from build123d import *

# Parameters (mm, degrees)
BOSS_EXTRUDE1_DEPTH  = 5
FILLET1_R            = 1
BOSS_EXTRUDE17_DEPTH = 7
CHAMFER1_SIZE        = 6
CHAMFER2_SIZE        = 6
CHAMFER3_SIZE        = 6


with BuildPart() as part:
    # Sketch2 → Boss-Extrude1 (new body)
    with BuildSketch(Plane.XY):
        with BuildLine():
            Line((-71.683238322, 36.264064839), (-71.683238322, -153.735935161))
            ThreePointArc((-71.683238322, -153.735935161), (-65.785654561, -167.973961861), (-51.547627861, -173.871545622))
            ThreePointArc((-51.547627861, -173.871545622), (38.452372139, -179.984063939), (128.452372139, -173.871545622))
            ThreePointArc((128.452372139, -173.871545622), (142.690398839, -167.973961861), (148.5879826, -153.735935161))
            Line((148.5879826, -153.735935161), (148.5879826, 36.264064839))
            ThreePointArc((148.5879826, 36.264064839), (146.404575746, 42.501121163), (140.807808283, 46.014571182))
            ThreePointArc((140.807808283, 46.014571182), (138.971586139, 46.086284232), (137.233469629, 45.489789872))
            ThreePointArc((137.233469629, 45.489789872), (38.452372139, 19.454880614), (-60.328725351, 45.489789872))
            ThreePointArc((-60.328725351, 45.489789872), (-62.066841861, 46.086284232), (-63.903064005, 46.014571182))
            ThreePointArc((-63.903064005, 46.014571182), (-69.499831468, 42.501121163), (-71.683238322, 36.264064839))
        make_face()
        with BuildLine():
            Line((-51.547627861, -162.258832658), (128.989007395, -162.258832658))
            ThreePointArc((128.989007395, -162.258832658), (131.022308029, -167.563941455), (126.782256855, -171.345535941))
            ThreePointArc((126.782256855, -171.345535941), (38.682041526, -176.831727196), (-49.421685934, -171.402229683))
            ThreePointArc((-49.421685934, -171.402229683), (-53.676249609, -167.572612121), (-51.547627861, -162.258832658))
        make_face(mode=Mode.SUBTRACT)
    extrude(amount=BOSS_EXTRUDE1_DEPTH)

    # Fillet1
    fillet1_edges = [part.edges().sort_by_distance(p)[0] for p in [
        (38.452372139, 19.454880614, 5),
        (38.452372139, -179.984063939, 0),
        (-65.785654561, -167.973961861, 0),
        (-71.683238322, -58.735935161, 0),
        (-69.499831468, 42.501121163, 0),
        (-62.066841861, 46.086284232, 0),
        (38.452372139, 19.454880614, 0),
        (138.971586139, 46.086284232, 0),
        (146.404575746, 42.501121163, 0),
        (-62.066841861, 46.086284232, 5),
        (-69.499831468, 42.501121163, 5),
        (128.452372139, -173.871545622, 2.5),
        (-51.547627861, -173.871545622, 2.5),
        (-71.683238322, -58.735935161, 5),
        (-65.785654561, -167.973961861, 5),
        (38.452372139, -179.984063939, 5),
        (142.690398839, -167.973961861, 5),
        (148.5879826, -58.735935161, 5),
        (146.404575746, 42.501121163, 5),
        (138.971586139, 46.086284232, 5),
        (148.5879826, -58.735935161, 0),
        (142.690398839, -167.973961861, 0),
    ]]
    fillet(fillet1_edges, radius=FILLET1_R)

    # Sketch3 → Boss-Extrude17 (add)
    with BuildSketch(Plane(origin=(0, 0, 0), x_dir=(-1, 0, 0), z_dir=(0, 0, -1))):
        Polygon((-60.193398692, -12.441134496), (-80.193398692, -23.98813988), (-80.193398692, -47.082150648), (-60.193398692, -58.629156031), (-40.193398692, -47.082150648), (-40.193398692, -23.98813988), align=None)
        Polygon((-39.260340262, -48.416474981), (-59.281974378, -59.975970827), (-59.281974378, -83.094962521), (-39.260340262, -94.654458367), (-19.238706146, -83.094962521), (-19.238706146, -59.975970827), align=None)
        Polygon((-59.655195417, -84.642570383), (-79.655195417, -96.189575767), (-79.655195417, -119.283586535), (-59.655195417, -130.830591919), (-39.655195417, -119.283586535), (-39.655195417, -96.189575767), align=None)
        Polygon((-18.449927197, -84.144928283), (-38.449927197, -95.691933667), (-38.449927197, -118.785944435), (-18.449927197, -130.332949819), (1.550072803, -118.785944435), (1.550072803, -95.691933667), align=None)
        Polygon((2.303708649, -48.596386935), (-17.696291351, -60.143392319), (-17.696291351, -83.237403087), (2.303708649, -94.78440847), (22.303708649, -83.237403087), (22.303708649, -60.143392319), align=None)
        Polygon((-80.491202658, -48.737511822), (-100.491202658, -60.284517205), (-100.491202658, -83.378527973), (-80.491202658, -94.925533357), (-60.491202658, -83.378527973), (-60.491202658, -60.284517205), align=None)
        Polygon((-18.755317237, -12.540627892), (-38.755317237, -24.087633275), (-38.755317237, -47.181644043), (-18.755317237, -58.728649427), (1.244682763, -47.181644043), (1.244682763, -24.087633275), align=None)
    extrude(amount=BOSS_EXTRUDE17_DEPTH)

    # Chamfer1
    chamfer1_edges = [part.edges().sort_by_distance(p)[0] for p in [
        (70.491202658, -54.511014514, -7),
        (90.491202658, -54.511014514, -7),
        (100.491202658, -71.831522589, -7),
        (90.491202658, -89.152030665, -7),
        (70.491202658, -89.152030665, -7),
        (60.491202658, -71.831522589, -7),
    ]]
    chamfer(chamfer1_edges, length=CHAMFER1_SIZE)

    # Chamfer2
    chamfer2_edges = [part.edges().sort_by_distance(p)[0] for p in [
        (-12.303708649, -54.369889627, -7),
        (7.696291351, -54.369889627, -7),
        (17.696291351, -71.690397703, -7),
        (7.696291351, -89.010905779, -7),
        (-12.303708649, -89.010905779, -7),
        (-22.303708649, -71.690397703, -7),
    ]]
    chamfer(chamfer2_edges, length=CHAMFER2_SIZE)

    # Chamfer3
    chamfer3_edges = [part.edges().sort_by_distance(p)[0] for p in [
        (50.193398692, -18.214637188, -7),
        (70.193398692, -18.214637188, -7),
        (80.193398692, -35.535145264, -7),
        (70.193398692, -52.855653339, -7),
        (50.193398692, -52.855653339, -7),
        (40.193398692, -35.535145264, -7),
        (29.249523204, -54.196222904, -7),
        (49.27115732, -54.196222904, -7),
        (59.281974378, -71.535466674, -7),
        (49.27115732, -88.874710444, -7),
        (29.249523204, -88.874710444, -7),
        (19.238706146, -71.535466674, -7),
        (49.655195417, -90.416073075, -7),
        (69.655195417, -90.416073075, -7),
        (79.655195417, -107.736581151, -7),
        (69.655195417, -125.057089227, -7),
        (49.655195417, -125.057089227, -7),
        (39.655195417, -107.736581151, -7),
        (8.449927197, -89.918430975, -7),
        (28.449927197, -89.918430975, -7),
        (38.449927197, -107.238939051, -7),
        (28.449927197, -124.559447127, -7),
        (8.449927197, -124.559447127, -7),
        (-1.550072803, -107.238939051, -7),
        (8.755317237, -18.314130583, -7),
        (28.755317237, -18.314130583, -7),
        (38.755317237, -35.634638659, -7),
        (28.755317237, -52.955146735, -7),
        (8.755317237, -52.955146735, -7),
        (-1.244682763, -35.634638659, -7),
    ]]
    chamfer(chamfer3_edges, length=CHAMFER3_SIZE)


solid = part.part
Build history of the part. All positions in model axes, mm. A direction names the side the tool comes from. Coordinates: 2 decimals unless noted, no trailing zeros. Order: outer loops, then holes, each group sorted by start corner. A loop starts at its lowest first (then second) coordinate and runs counter-clockwise, first axis right, second up. Notation, with made-up numbers: (-19, 8.5) - (-12, 8.5) arc R27 ccw to (-12, 38.5) - close; hole circle Ø5 at (86, 58). An arc over 180 degrees is marked (long way). Write each question's results on one line, items separated by ' | '. Start each with the question number.
Item 1: Band-saw the part on B-B on z = -3.5. State how many separate pieces and enclosed holes the cut face has, and give its area (3 significant figures).
Item 2: Flat gauge pins, fed straight in: pin 1 (5 mm diameter, centred on x = -24.5, z = 1.5, fed in from +Y); pin 2 (3 mm diameter, centred on y = -30, z = -4, fed in from +X); pin 3 (3 mm diameter, centred on y = -2, z = 0.5, fed in from +X); pin 4 (0.5 mm diameter, centred on y = -38, z = -0.5, fed in from -X). Where does each tip first touch, or does it go through?
Item 3: Wall check: probe 1 along X at (y, z) = (-75.5, -4); probe 2 along Z at (x, y) = (102, -87.5); probe 3 along X at (y, z) = (-53.5, -4). Give the ranges that are in metal, low to high. Write a range as [from, to].
Item 4: Band-saw the part on A-A on y = -71. Write the cut outline in (x, z), and give its area (3 significant figures).
Item 5: Mould opens along Y. For faces 4 (the face through (49.4, -88.8, -0.5)), 5 (the face through (19, -35, -7)), 6 (the face through (68.532, -20.768, -4.042)) say: released by +Y, released by -Y, zero draft, split by the parting line, or undercut.
Item 6: Tool access for faces 1 (the face through (77.151, -35.373, -4.042)), 2 (the face through (42.697, -107.898, -4.042)), 3 (the face through (29.109, -54.277, -0.493)): list every direction of +Z, -Z, +X, -X, +Y, -Y with a clear straight run to the whole face (end or side of a thin tool).
Numbers:
1) separate pieces: 7 | enclosed holes: 0 | area: 7,430 mm^2
2) pin 1: y = 30.44 | pin 2: x = 78.69 | pin 3: x = 148.59 | pin 4: x = -1.24
3) probe 1: [-19.3, 14.7], [22.24, 56.28], [63.49, 97.49] | probe 2: [0, 5] | probe 3: [-4.8, 0.19], [15.7, 21.81], [36.46, 42.07], [57.31, 63.08], [78.24, 82.74]
4) outline: (-71.68, 1) arc R1 ccw to (-70.68, 0) - (-22.3, 0) - (-22.3, -1) - (-16.3, -7) - (11.7, -7) - (17.7, -1) - (17.7, 0) - (19.24, 0) - (19.24, -1) - (25.24, -7) - (53.28, -7) - (59.28, -1) - (59.28, 0) - (60.49, 0) - (60.49, -1) - (66.49, -7) - (94.49, -7) - (100.49, -1) - (100.49, 0) - (147.59, 0) arc R1 ccw to (148.59, 1) - (148.59, 4) arc R1 ccw to (147.59, 5) - (-70.68, 5) arc R1 ccw to (-71.68, 4) - close | area: 1,830 mm^2
5) face 4: undercut | face 5: zero draft | face 6: released by +Y
6) face 1: -Z, +X, +Y | face 2: -Z, -Y | face 3: -Z
